from build123d import *

# Parameters (mm, degrees)
F0_W      = 163.6395
F0_H      = 54.1782
F1_DEPTH  = 3.175
F2_W      = 9.398
F2_H      = 9.398
F3_DEPTH  = 11.43
F4_W      = 9.398
F4_H      = 9.398
F5_DEPTH  = 10.16
F6_R      = 2.54
F7_R      = 2.54
F8_W      = 6.223
F8_H      = 6.223
F9_DEPTH  = 8.255
F10_R     = 2.032
F12_DEPTH = 25.4
F13_R     = 12.7
F15_DEPTH = 6.35


# Not quite as in the source:
# - a feature names something its author has since deleted; it is built from what else it names


with BuildPart() as f1:
    # F0 (on Top) → F1 (new body)
    with BuildSketch(Plane.XY):
        with Locations((72.10425, -26.6827)):
            Rectangle(F0_W, F0_H)
    extrude(amount=-F1_DEPTH)

    # F2 (on Top) → F3 (join)
    with BuildSketch(Plane.XY):
        with Locations((14.0335, -13.9446)):
            Rectangle(F2_W, F2_H)
        with Locations((39.3065, -13.9446)):
            Rectangle(F2_W, F2_H)
        with Locations((62.9285, -13.9446)):
            Rectangle(F2_W, F2_H)
        with Locations((85.5345, -13.9446)):
            Rectangle(F2_W, F2_H)
        with Locations((106.9975, -13.9446)):
            Rectangle(F2_W, F2_H)
        with Locations((127.3175, -13.9446)):
            Rectangle(F2_W, F2_H)
    extrude(amount=F3_DEPTH)

    # F4 (on face) → F5 (join)
    with BuildSketch(Plane.XY):
        with Locations((101.6635, -39.3446)):
            Rectangle(F4_W, F4_H)
        with Locations((138.7475, -39.3446)):
            Rectangle(F4_W, F4_H)
        with Locations((119.6975, -39.3446)):
            Rectangle(F4_W, F4_H)
        with Locations((83.8835, -39.3446)):
            Rectangle(F4_W, F4_H)
        with Locations((66.1035, -39.3446)):
            Rectangle(F4_W, F4_H)
    extrude(amount=F5_DEPTH)

    # F6
    f6_edges = [f1.edges().sort_by_distance(p)[0] for p in [
        (14.0335, -9.2456, 11.43),
        (9.3345, -13.9446, 11.43),
        (14.0335, -18.6436, 11.43),
        (18.7325, -13.9446, 11.43),
        (44.0055, -13.9446, 11.43),
        (39.3065, -9.2456, 11.43),
        (34.6075, -13.9446, 11.43),
        (39.3065, -18.6436, 11.43),
        (67.6275, -13.9446, 11.43),
        (62.9285, -9.2456, 11.43),
        (58.2295, -13.9446, 11.43),
        (62.9285, -18.6436, 11.43),
        (90.2335, -13.9446, 11.43),
        (85.5345, -9.2456, 11.43),
        (80.8355, -13.9446, 11.43),
        (85.5345, -18.6436, 11.43),
        (111.6965, -13.9446, 11.43),
        (106.9975, -9.2456, 11.43),
        (102.2985, -13.9446, 11.43),
        (106.9975, -18.6436, 11.43),
        (132.0165, -13.9446, 11.43),
        (127.3175, -9.2456, 11.43),
        (122.6185, -13.9446, 11.43),
        (127.3175, -18.6436, 11.43),
    ]]
    fillet(f6_edges, radius=F6_R)

    # F7
    f7_edges = [f1.edges().sort_by_distance(p)[0] for p in [
        (66.1035, -34.6456, 10.16),
        (61.4045, -39.3446, 10.16),
        (66.1035, -44.0436, 10.16),
        (70.8025, -39.3446, 10.16),
        (83.8835, -34.6456, 10.16),
        (79.1845, -39.3446, 10.16),
        (83.8835, -44.0436, 10.16),
        (88.5825, -39.3446, 10.16),
        (101.6635, -34.6456, 10.16),
        (96.9645, -39.3446, 10.16),
        (101.6635, -44.0436, 10.16),
        (106.3625, -39.3446, 10.16),
        (119.6975, -34.6456, 10.16),
        (114.9985, -39.3446, 10.16),
        (119.6975, -44.0436, 10.16),
        (124.3965, -39.3446, 10.16),
        (138.7475, -34.6456, 10.16),
        (134.0485, -39.3446, 10.16),
        (138.7475, -44.0436, 10.16),
        (143.4465, -39.3446, 10.16),
    ]]
    fillet(f7_edges, radius=F7_R)

    # F8 (on face) → F9 (join)
    with BuildSketch(Plane.XY):
        with Locations((50.8635, -39.3446)):
            Rectangle(F8_W, F8_H)
        with Locations((38.1635, -39.3446)):
            Rectangle(F8_W, F8_H)
        with Locations((25.4635, -39.3446)):
            Rectangle(F8_W, F8_H)
        with Locations((12.7635, -39.3446)):
            Rectangle(F8_W, F8_H)
        with Locations((0.0635, -39.3446)):
            Rectangle(F8_W, F8_H)
    extrude(amount=F9_DEPTH)

    # F10
    f10_edges = [f1.edges().sort_by_distance(p)[0] for p in [
        (50.8635, -36.2331, 8.255),
        (47.752, -39.3446, 8.255),
        (50.8635, -42.4561, 8.255),
        (53.975, -39.3446, 8.255),
        (41.275, -39.3446, 8.255),
        (38.1635, -36.2331, 8.255),
        (35.052, -39.3446, 8.255),
        (38.1635, -42.4561, 8.255),
        (28.575, -39.3446, 8.255),
        (25.4635, -36.2331, 8.255),
        (22.352, -39.3446, 8.255),
        (25.4635, -42.4561, 8.255),
        (15.875, -39.3446, 8.255),
        (12.7635, -36.2331, 8.255),
        (9.652, -39.3446, 8.255),
        (12.7635, -42.4561, 8.255),
        (3.175, -39.3446, 8.255),
        (0.0635, -36.2331, 8.255),
        (-3.048, -39.3446, 8.255),
        (0.0635, -42.4561, 8.255),
    ]]
    fillet(f10_edges, radius=F10_R)

    # F11 (on face) → F12 (cut)
    with BuildSketch(Plane.XY):
        Polygon((-9.7155, -36.2331), (2.9845, 0.4064), (-15.3606878594, 6.279731635), align=None)
        Polygon((160.9365438023, 5.6682056747), (138.3665, 0.4064), (153.924, -34.6456), align=None)
    extrude(amount=-F12_DEPTH, mode=Mode.SUBTRACT)

    # F13
    f13_edges = [f1.edges().sort_by_distance(p)[0] for p in [
        (2.9845, 0.4064, -1.5875),
        (-9.7155, -36.2331, -1.5875),
        (-9.7155, -53.7718, -1.5875),
        (153.924, -53.7718, -1.5875),
        (153.924, -34.6456, -1.5875),
        (138.3665, 0.4064, -1.5875),
    ]]
    fillet(f13_edges, radius=F13_R)

    # F14 (on face) → F15 (join)
    with BuildSketch(Plane(origin=(0, 0, -3.175), x_dir=(1, 0, 0), z_dir=(0, 0, -1))):
        with BuildLine():
            Line((141.224, 56.9468), (2.9845, 56.9468))
            ThreePointArc((2.9845, 56.9468), (-8.2408201513, 52.2971201513), (-12.8905, 41.0718))
            Line((-12.8905, 41.0718), (-12.8905, 38.3717247645))
            ThreePointArc((-12.8905, 38.3717247645), (-12.6700922272, 35.7355595192), (-12.0149891716, 33.172595069))
            Line((-12.0149891716, 33.172595069), (-2.9757778148, 7.0944703045))
            ThreePointArc((-2.9757778148, 7.0944703045), (2.8182933575, -0.6399186418), (12.0237113568, -3.5814))
            Line((12.0237113568, -3.5814), (130.1085556284, -3.5814))
            ThreePointArc((130.1085556284, -3.5814), (138.7624146724, -1.0152823214), (144.6185640244, 5.8534694619))
            Line((144.6185640244, 5.8534694619), (155.734008396, 30.8972461686))
            ThreePointArc((155.734008396, 30.8972461686), (156.754003353, 34.0457781807), (157.099, 37.3373767067))
            Line((157.099, 37.3373767067), (157.099, 41.0718))
            ThreePointArc((157.099, 41.0718), (152.4493201513, 52.2971201513), (141.224, 56.9468))
        make_face()
        with BuildLine():
            Line((152.8320067168, 32.1852722762), (141.7165623452, 7.1414955695))
            ThreePointArc((141.7165623452, 7.1414955695), (137.0316428636, 1.6464941428), (130.1085556284, -0.4064))
            Line((130.1085556284, -0.4064), (12.0237113568, -0.4064))
            ThreePointArc((12.0237113568, -0.4064), (4.6593769574, 1.9467850865), (0.0241200196, 8.1342962436))
            Line((0.0241200196, 8.1342962436), (-9.0150913373, 34.2124210081))
            ThreePointArc((-9.0150913373, 34.2124210081), (-9.5391737818, 36.2627925683), (-9.7155, 38.3717247645))
            Line((-9.7155, 38.3717247645), (-9.7155, 41.0718))
            ThreePointArc((-9.7155, 41.0718), (-5.9957561211, 50.0520561211), (2.9845, 53.7718))
            Line((2.9845, 53.7718), (141.224, 53.7718))
            ThreePointArc((141.224, 53.7718), (150.2042561211, 50.0520561211), (153.924, 41.0718))
            Line((153.924, 41.0718), (153.924, 37.3373767067))
            ThreePointArc((153.924, 37.3373767067), (153.6480026824, 34.7040978859), (152.8320067168, 32.1852722762))
        make_face(mode=Mode.SUBTRACT)
    extrude(amount=-F15_DEPTH)


solid = f1.part
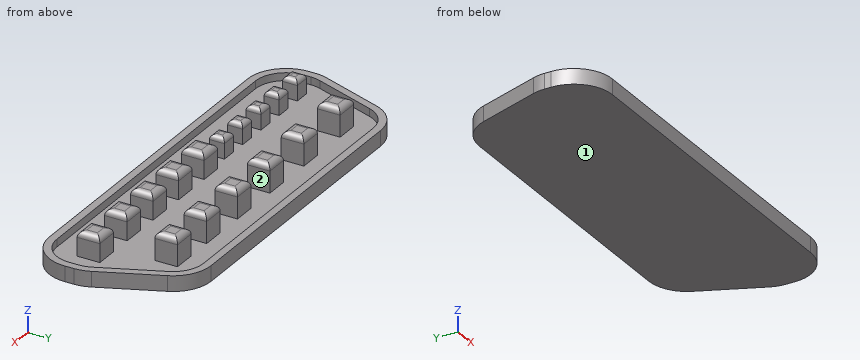
Verification items for the finished model (mm, model axes). Face numbers are marked on the shaded views. Give positions to 0.01 mm unless a question says otherwise; leave off trailing zeros. Write each loop counter-clockwise with the first axis right and the second up, starting at its lowest first coordinate (ties: lowest second). Pieces come first, ordered by that corner, then holes. Notation, with made-up numbers: (66.25, -25.75) - (113.25, -25.75) arc R12 cw to (113.25, -5.75) - close; hole circle Ø7 at (-15.75, -3). An arc over 180 degrees is marked (long way). Answer as CSV lines item,"result". Start each with the question number.
1. Sectioned sample at B-B (y = -28.5). Record the boundary of the cut face in (x, z) (3 decimals).
2. Draft check along X on the marked faces 1 and 2. Enter one of: pulls with the +X half, pulls with the -X half, needs draft (parallel to the pull), parting line crosses it, or undercut.
3. Depth check by flat-ended pin: pin 1 (7 mm diameter, centred on y = -14, z = 6, fed in from -X); pin 2 (4.5 mm diameter, centred on x = 12.5, z = 5.5, fed in from -Y); pin 3 (4.5 mm diameter, centred on y = -13.5, z = 4.5, fed in from -X). Enter the tip coordinate at first touch or a pass-through.
4. Sectioned sample at C-C (y = -22). Record the boundary of the cut face in (x, z) (3 decimals), then the cut area to 3 significant figures.
5. Thickness scan on line 1 (Y direction, x = 102, z = 0.25); line 2 (Y direction, x = 110, z = 2.5); line 3 (X direction, y = -14, z = 7.5). Record the ranges inside material, lowest first.
Derived:
1,outline,"(-10.395, -3.175) - (154.67, -3.175) - (154.67, 3.175) - (151.196, 3.175) - (151.196, 0) - (-7.035, 0) - (-7.035, 3.175) - (-10.395, 3.175) - close"
2,face 1,"needs draft"
2,face 2,"undercut"
3,pin 1,"x = -6.09"
3,pin 2,"y = -42.46"
3,pin 3,"x = -5.83"
4,outline,"(-8.142, -3.175) - (151.785, -3.175) - (151.785, 3.175) - (148.311, 3.175) - (148.311, 0) - (-4.782, 0) - (-4.782, 3.175) - (-8.142, 3.175) - close"
4,area,"529 mm²"
5,line 1,"-56.95 to -53.77, -44.04 to -34.65, 0.41 to 3.58"
5,line 2,"-56.95 to -53.77, -18.64 to -9.25, 0.41 to 3.58"
5,line 3,"9.33 to 18.73, 34.61 to 44.01, 58.23 to 67.63, 80.84 to 90.23, 102.3 to 111.7, 122.62 to 132.02"
